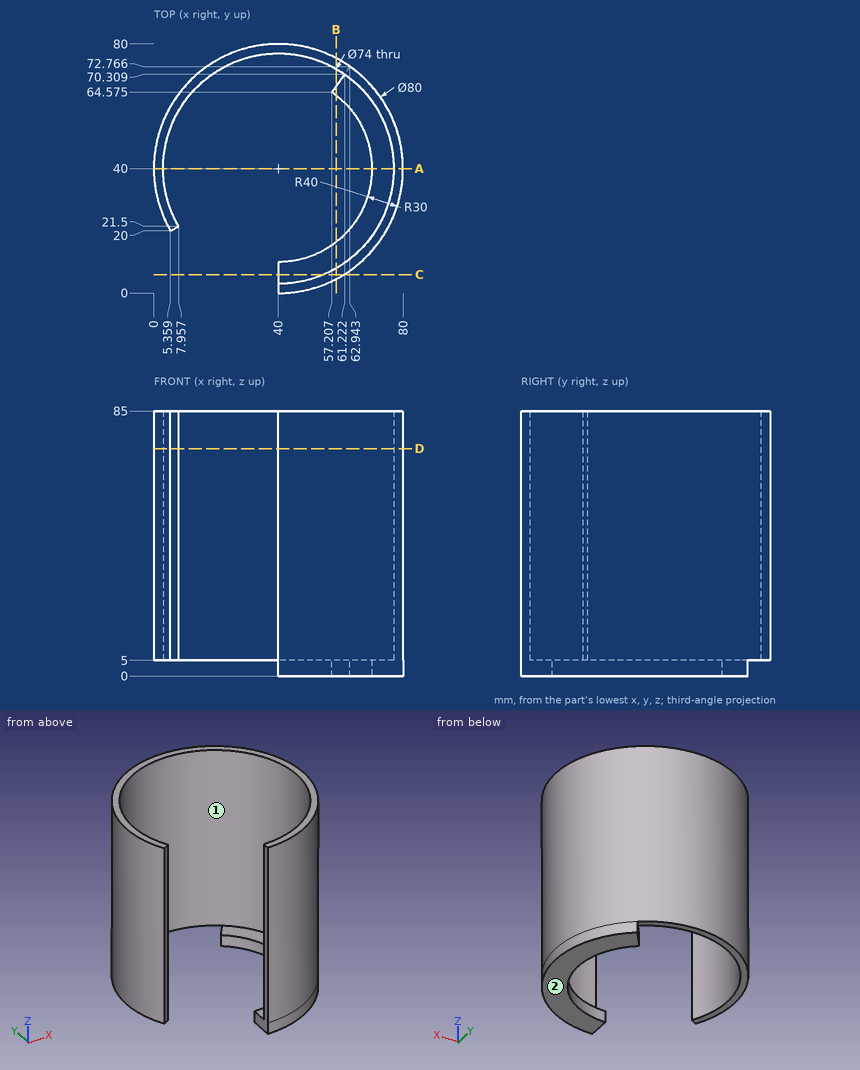
The figure shows three views and two pictorial views of one solid part (mm, origin at its lowest corner). Answer the questions. Give positions to 0.01 mm unless a question says otherwise; leave off trailing zeros. Order: outer loops, then holes, each group sorted by start corner. A loop starts at its lowest first (then second) coordinate and runs counter-clockwise, first axis right, second up. Notation, with made-up numbers: (10.25, 53.5) -> (41.25, 53.5) arc R27 cw to (41.25, 76.5) -> close; hole circle Ø11 at (-12, 67). An arc over 180 degrees is marked (long way). Write each question's results on one line, items separated by ' | '.
Q1. Each of these flat-tipped pins is pushed along its axis until it touches: P1, Ø1, axis at x = 64.5, z = 75.5, coming from the -Y side; P2, Ø2, axis at y = 15.5, z = 73.5, coming from the +X side; P3, Ø1, axis at y = 50.5, z = 28.5, coming from the +X side. Where does it stop, or does it pass through?
Checked values:
P1: stops at y = 8 | P2: stops at x = 72.37 | P3: stops at x = 78.73
Q2. The part is cut by section B-B, the plane x = 58.5. Give the vertices of the cut face in (y, z) (1 decimal).
Checked values:
outline: (4.5, 0) -> (16.4, 0) -> (16.4, 5) -> (8, 5) -> (8, 85) -> (4.5, 85) -> close; (63.6, 0) -> (66.4, 0) -> (66.4, 5) -> (63.6, 5) -> close; (72, 5) -> (75.5, 5) -> (75.5, 85) -> (72, 85) -> close
Q3. The part is cut by section D-D, the plane z = 73. Give the vertices of the cut face in (x, y).
Checked values:
outline: (5.36, 20) -> (7.96, 21.5) arc R37 cw (long way) to (40, 3) -> (40, 0) arc R40 ccw (long way) to start
Q4. The part is cut by section A-A, the plane y = 40. Give the vertices of the cut face in (x, z).
Checked values:
outline: (0, 5) -> (3, 5) -> (3, 85) -> (0, 85) -> close; (70, 0) -> (80, 0) -> (80, 85) -> (77, 85) -> (77, 5) -> (70, 5) -> close
Q5. Determine the mould class of the marked faces 1 and 2 for opening direction X: pulls with the +X half, pulls with the -X half, needs draft (parallel to the pull), parting line crosses it, or undercut.
Checked values:
face 1: undercut | face 2: needs draft
Q6. The part is cut by section C-C, the plane y = 6. Give the vertices of the cut face in (x, z) (1 decimal).
Checked values:
outline: (40, 0) -> (61.1, 0) -> (61.1, 85) -> (54.6, 85) -> (54.6, 5) -> (40, 5) -> close
Q7. Straight lines are drawn through the part: probe 1 along X at (y, z) = (40, 55); probe 2 along Z at (x, y) = (61, 15.5); probe 3 along Y at (x, z) = (39.5, 24.5). For each, find the intervals that lie inside material, in ascending order. Write a range as from..to.
Checked values:
probe 1: x = 0..3, 77..80 | probe 2: z = 0..5 | probe 3: y = 77..80
